from build123d import *

# Parameters (mm, degrees)
CROQUIS1_R              = 3.175
SALIENTE_EXTRUIR1_DEPTH = 3.1242


with BuildPart() as part:
    # Croquis1 → Saliente-Extruir1 (new body)
    with BuildSketch(Plane.XY):
        with BuildLine():
            Line((-9.525, 0), (-9.525, 33.3375))
            ThreePointArc((-9.525, 33.3375), (0, 42.8625), (9.525, 33.3375))
            Line((9.525, 33.3375), (9.525, 0))
            ThreePointArc((9.525, 0), (0, -9.525), (-9.525, 0))
        make_face()
        Circle(CROQUIS1_R, mode=Mode.SUBTRACT)
        with BuildLine():
            Line((-2.032, 6.35), (-2.032, 12.7))
            ThreePointArc((-2.032, 12.7), (0, 14.732), (2.032, 12.7))
            Line((2.032, 12.7), (2.032, 6.35))
            ThreePointArc((2.032, 6.35), (0, 4.318), (-2.032, 6.35))
        make_face(mode=Mode.SUBTRACT)
        with BuildLine():
            Line((6.35, 33.3375), (6.35, 26.9875))
            ThreePointArc((6.35, 26.9875), (0, 20.6375), (-6.35, 26.9875))
            Line((-6.35, 26.9875), (-6.35, 33.3375))
            ThreePointArc((-6.35, 33.3375), (0, 39.6875), (6.35, 33.3375))
        make_face(mode=Mode.SUBTRACT)
    extrude(amount=SALIENTE_EXTRUIR1_DEPTH)


solid = part.part
The listing builds one solid part. Answer for the finished solid, in the listing's coordinates (mm). A direction names the side the tool comes from. Round coordinates to 2 decimals unless told otherwise and drop trailing zeros. Write each loop counter-clockwise with the first axis right and the second up, starting at its lowest first coordinate (ties: lowest second). Pieces come first, ordered by that corner, then holes. Notation, with made-up numbers: M -8.5,-22 L 21.5,-22 A20 ccw 21.5,-16 Z; hole C 44.5,80 d10. An arc over 180 degrees is marked long. Write each question's results on one line, items separated by ' | '. Start each with the question number.
Item 1: Which of the six approach directions +Z, -Z, +X, -X, +Y, -Y give full straight-line access (tool end or side, diameter ignored) to faces 1 (the flat face through (0, 17, 0)), 2 (the cylindrical face through (0.04, 4.32, 1.54))?
Item 2: Find section C-C on x = 5. Write down the section's boundary in (y, z).
Item 3: The mould has two halves that part along Y. Classify faces 3 (the flat face through (9.525, 17, 2)), 4 (the cylindrical face through (-0.21, 42.86, 1.54)), 5 (the flat face through (6.35, 30, 2)): +Y half, -Y half, draft (parallel to the pull), parting line (faces both ways), or undercut.
Item 4: Given pin 1 Ø5 at (x, y) = (-5, 29) entering from +Z, flat-ended and moving along its own axis, determine where the tip first touches the part or whether it passes through.
Item 5: Find section A-A on z = 0.8. Give the number of separate pieces and of enclosed holes in the cut face, and give its area (3 significant figures).
Item 6: Find section D-D on x = 0. Write down the section's boundary in (y, z) (1 decimal).
Item 7: Find section B-B on y = 30.5. Write down the section's boundary in (x, z) (3 decimals).
Item 8: Straight lines are drawn through the part: probe 1 along Y at (x, z) = (0, 1.25) (1 decimal); probe 2 along Y at (x, z) = (-1.5, 1.45); probe 3 along X at (y, z) = (8, 1.85) (3 decimals). For each, find the intervals that lie inside material, in ascending order.
Answer block:
1) face 1: -Z, +X, -X, +Y, -Y | face 2: +Z, -Z
2) outline: M -8.11,0 L 23.07,0 L 23.07,3.12 L -8.11,3.12 Z; M 37.25,0 L 41.44,0 L 41.44,3.12 L 37.25,3.12 Z
3) face 3: draft | face 4: +Y half | face 5: undercut
4) pin 1: stops at z = 3.12
5) separate pieces: 1 | enclosed holes: 3 | area: 642 mm²
6) outline: M -9.5,0 L -3.2,0 L -3.2,3.1 L -9.5,3.1 Z; M 3.2,0 L 4.3,0 L 4.3,3.1 L 3.2,3.1 Z; M 14.7,0 L 20.6,0 L 20.6,3.1 L 14.7,3.1 Z; M 39.7,0 L 42.9,0 L 42.9,3.1 L 39.7,3.1 Z
7) outline: M -9.525,0 L -6.35,0 L -6.35,3.124 L -9.525,3.124 Z; M 6.35,0 L 9.525,0 L 9.525,3.124 L 6.35,3.124 Z
8) probe 1: y = -9.5 to -3.2, 3.2 to 4.3, 14.7 to 20.6, 39.7 to 42.9 | probe 2: y = -9.41 to -2.8, 2.8 to 4.98, 14.07 to 20.82, 39.51 to 42.74 | probe 3: x = -9.525 to -2.032, 2.032 to 9.525
